Autodesk Inventor part; units mm, degrees
ref_plane "YZ Plane" through (0, 0, 0) normal (1, 0, 0) x (0, 1, 0)
ref_plane "XZ Plane" through (0, 0, 0) normal (0, 1, 0) x (-1, 0, 0)
ref_plane "XY Plane" through (0, 0, 0) normal (0, 0, 1) x (1, 0, 0)
sketch "Sketch1" plane through (0, 0, 0) normal (0, 0, 1) x (1, 0, 0)
  line L0 (-15.5, 11) -> (14, 11)
  line L1 (14, 11) -> (14, -10)
  line L2 (14, -10) -> (-15.5, -10)
  line L3 (-15.5, -10) -> (-15.5, 11)
  point P0 (0, 0)
  dimension "d0" = 29.5
  dimension "d1" = 21
  dimension "d2" = 10
  dimension "d3" = 14
extrude "Extrusion1" add sketch "Sketch1" against normal blind 3.55
sketch "Sketch2" plane through (0, 0, 0) normal (0, 0, 1) x (1, 0, 0)
  line L0 (-15.5, 11) -> (14, 11)
  line L1 (14, 11) -> (14, 0)
  line L2 (14, 0) -> (-15.5, 0)
  line L3 (-15.5, 0) -> (-15.5, 11)
  line L4 (14, 11) -> (-15.5, 11)
  point P0 (0, 0)
  dimension "d6" = 29.5
  dimension "d8" = 0
  dimension "d27" = 0
  dimension "d77" = 14
extrude "Extrusion2" add sketch "Sketch2" along normal blind 1.5
sketch "Sketch3" plane through (0, 0, 1.5) normal (0, 0, 1) x (1, 0, 0)
  line L0 (-15.5, 0) -> (14, 0)
  line L1 (14, 11) -> (-15.5, 11)
  point P0 (0, 0)
  point P1 (0, 5.5)
  dimension "d12" = 0
  dimension "d28" = 11
  dimension "d29" = 5.5
sketch "Sketch5" plane through (0, 0, -3.55) normal (0, 0, -1) x (-1, 0, 0)
  line L0 (15.5, -10) -> (15.5, 11)
  line L1 (-14, 0) -> (15.5, 0)
  line L2 (-14, -10) -> (15.5, -10)
  line L3 (-14, -10) -> (-14, 0)
  point P0 (0, 0)
  point P1 (0, -4.5)
  dimension "d19" = 4.5
  dimension "d78" = 14
hole "Hole1" at (0, -4.5, -3.55) direction (0, 0, 1) diameter 4.5 end through all counterbore diameter 7.94 counterbore depth 0.5
hole "Hole2" at (0, 5.5, 1.5) direction (0, 0, -1) diameter 4.5 end through all counterbore diameter 8 counterbore depth 1.25
sketch "Sketch6" plane through (0, 0, -3.55) normal (0, 0, -1) x (-1, 0, 0)
  line L0 (5.498, 5.5) -> (4.502, 5.5) construction
  line L1 (5.498, 6.55) -> (4.502, 6.55)
  line L2 (4.502, 4.45) -> (5.498, 4.45)
  arc A0 (5.498, 4.45) -> (5.498, 6.55) centre (5.498, 5.5) ccw
  arc A1 (4.502, 6.55) -> (4.502, 4.45) centre (4.502, 5.5) ccw
  point P0 (0, 0)
  point P1 (0, 5.5)
  point P2 (-5, 5.5)
  point P3 (5, 5.5)
  dimension "d37" = 0
  dimension "d38" = 5.5
  dimension "d39" = 0
  dimension "d40" = 5
  dimension "d41" = 0
  dimension "d42" = 5
  dimension "d58" = 1.05
  dimension "d60" = 0.996
hole "Hole3" at (5, 5.5, -3.55) direction (0, 0, 1) diameter 2.1 depth 2
sketch "Sketch8" plane through (0, 0, 0) normal (0, 0, 1) x (1, 0, 0)
  circle A0 centre (0, -4.5) radius 3.5
  circle A1 centre (0, -4.5) radius 2.25
  point P0 (0, 0)
  dimension "d53" = 0
  dimension "d54" = 0
  dimension "d55" = 7
extrude "Extrusion3" cut sketch "Sketch8" against normal blind 0.5
extrude "Extrusion4" cut sketch "Sketch6" against normal blind 2.1
chamfer "Chamfer3" distance 1 angle 45 4 edges at (14, 11, -1.025) (-15.5, 11, -1.025) (14, -10, -1.775) (-15.5, -10, -1.775)
sketch "Sketch9" plane through (-14.5, 11, 1.5) normal (0, 1, 0) x (1, 0, 0)
  circle A0 centre (14.5, 17.4) radius 12.7
  line L0 (27.5, 0) -> (0, 0)
  point P0 (14.5, 1.5)
  point P1 (30, 0)
  point P2 (0.5, 0)
  dimension "d72" = 0
  dimension "d73" = 25.4
  dimension "d74" = 17.4
extrude "Extrusion5" cut sketch "Sketch9" against normal up to surface (21 mm away)
sketch "Sketch10" plane through (-14.5, 11, 1.5) normal (0, 1, 0) x (1, 0, 0)
  circle A0 centre (23.017, -3.75) radius 5.25
  line L0 (27.5, 0) -> (0, 0)
  point P0 (14.5, 1.5)
  point P1 (19.3428, 0)
  point P2 (26.6912, 0)
  dimension "d79" = 10.5
  dimension "d82" = 3.75
  dimension "d83" = 8.517
extrude "Extrusion6" [suppressed]
sketch "Sketch11" plane through (0, 0, 1.5) normal (0, 0, 1) x (1, 0, 0)
  line L0 (5, 11) -> (14, 11)
  line L1 (14, 11) -> (14, 2)
  line L2 (14, 2) -> (7, 2)
  line L3 (5, 4) -> (5, 11)
  line L4 (13, 11) -> (-14.5, 11)
  line L5 (14, 0) -> (14, 10)
  line L6 (-15.5, 0) -> (14, 0)
  arc A0 (5, 4) -> (7, 2) centre (7, 4) ccw
  point P0 (0, 0)
  point P1 (5, 2)
  point P2 (4.8428, 11)
  point P3 (12.1912, 0)
  dimension "d86" = 0
  dimension "d87" = 0
  dimension "d88" = 9
  dimension "d89" = 2
  dimension "d94" = 2
extrude "Extrusion7" cut sketch "Sketch11" against normal blind 1.5
equation "\"d6\" = d0"
properties part number "rd-mount"
The listing builds one solid part. Answer for the finished solid, in the listing's coordinates (mm). A direction names the side the tool comes from. Coordinates: 2 decimals unless noted, no trailing zeros. Write each loop counter-clockwise with the first axis right and the second up, starting at its lowest first coordinate (ties: lowest second). Pieces come first, ordered by that corner, then holes. Notation, with made-up numbers: (70.5, 19) - (103.5, 19) arc R13 cw to (103.5, 23) - close; hole circle Ø2 at (-39.5, 2.25). An arc over 180 degrees is marked (long way). One line per item, written item: value.
1) Each of these flat-tipped pins is pushed along its axis until it touches: pin 1 Ø0.8 at (x, z) = (12, 0.5) entering from +Y; pin 2 Ø6 at (x, y) = (9, -4) entering from +Z; pin 3 Ø6.5 at (x, y) = (-2, -5.5) entering from -Z; pin 4 Ø1 at (x, y) = (-1.5, 2.5) entering from +Z. Where does it stop, or does it pass through?
Geometry check:
pin 1: stops at y = 2
pin 2: stops at z = 0
pin 3: stops at z = -3.55
pin 4: stops at z = 0.25
2) Find section C-C (z = -2.25). Give the vertices of the cut face in (x, y), and give its area (3 significant figures).
Geometry check:
outline: (-15.5, -9) - (-14.5, -10) - (13, -10) - (14, -9) - (14, 10) - (13, 11) - (-14.5, 11) - (-15.5, 10) - close; hole (-5.5, 4.45) - (-4.5, 4.45) arc R1.05 ccw to (-4.5, 6.55) - (-5.5, 6.55) arc R1.05 ccw to start; hole circle Ø4.5 at (0, -4.5); hole circle Ø4.5 at (0, 5.5); hole circle Ø2.1 at (5, 5.5)
area: 577 mm2
3) Find section B-B (x = 0). Give the vertices of the cut face in (y, z).
Geometry check:
outline: (-10, -3.2) - (-8.47, -3.2) - (-8.47, -3.05) - (-6.75, -3.05) - (-6.75, -0.5) - (-8, -0.5) - (-8, 0) - (-10, 0) - close; (-2.25, -3.05) - (-0.53, -3.05) - (-0.53, -3.2) - (3.25, -3.2) - (3.25, 0.25) - (1.5, 0.25) - (1.5, 1.5) - (0, 1.5) - (0, 0) - (-1, 0) - (-1, -0.5) - (-2.25, -0.5) - close; (7.75, -3.2) - (11, -3.2) - (11, 1.5) - (9.5, 1.5) - (9.5, 0.25) - (7.75, 0.25) - close
4) Find section D-D (y = 5.5). Give the vertices of the cut face in (x, z).
Geometry check:
outline: (-15.5, -3.55) - (-6.55, -3.55) - (-6.55, -1.45) - (-3.45, -1.45) - (-3.45, -3.55) - (-2.96, -3.55) arc R12.7 cw to (-2.25, -3.4) - (-2.25, 0.25) - (-4, 0.25) - (-4, 1.5) - (-15.5, 1.5) - close; (2.25, -3.4) arc R12.7 cw to (2.96, -3.55) - (3.95, -3.55) - (3.95, -1.55) - (6.05, -1.55) - (6.05, -3.55) - (14, -3.55) - (14, 0) - (5, 0) - (5, 1.5) - (4, 1.5) - (4, 0.25) - (2.25, 0.25) - close
5) Find section A-A (y = -4.5). Give the vertices of the cut face in (x, z).
Geometry check:
outline: (-15.5, -3.55) - (-3.97, -3.55) - (-3.97, -3.05) - (-2.25, -3.05) - (-2.25, -0.5) - (-3.5, -0.5) - (-3.5, 0) - (-15.5, 0) - close; (2.25, -3.05) - (3.97, -3.05) - (3.97, -3.55) - (14, -3.55) - (14, 0) - (3.5, 0) - (3.5, -0.5) - (2.25, -0.5) - close
6) Consider line 1 along Y through (x, z) = (0, -0.3); line 2 along Y through (x, z) = (0, 0.6); line 3 along X through (y, z) = (-4.5, -1.7). Determine where each line is inside the solid, lowest interval first. Write a range as from..to.
Geometry check:
line 1: y = -10..-8, -1..3.25, 7.75..11
line 2: y = 0..1.5, 9.5..11
line 3: x = -15.5..-2.25, 2.25..14
7) For a pull along Y with two mould halves and no side action, classify faces 1 (the flat face through (-5, 6.55, -3)), 2 (the flat face through (-4.2, 5.6, 1.5)), 3 (the flat face through (13.5, -9.5, -1.8)) as pulls with the +Y half, pulls with the -Y half, needs draft (parallel to the pull), parting line crosses it, or undercut.
Geometry check:
face 1: undercut
face 2: needs draft
face 3: pulls with the -Y half
8) A tool of negligible diameter and unlimited length cuts with its end or side. For faces 4 (the cylindrical face through (-6.548, 5.477, -2.515)), 5 (the flat face through (2, 4, 0.25)), 6 (the flat face through (11, 2, 1)), from which of +Z, -Z, +X, -X, +Y, -Y can it reach the whole face along a straight path? Write none if from no direction.
Geometry check:
face 4: -Z
face 5: +Z
face 6: +Z, +X, +Y
